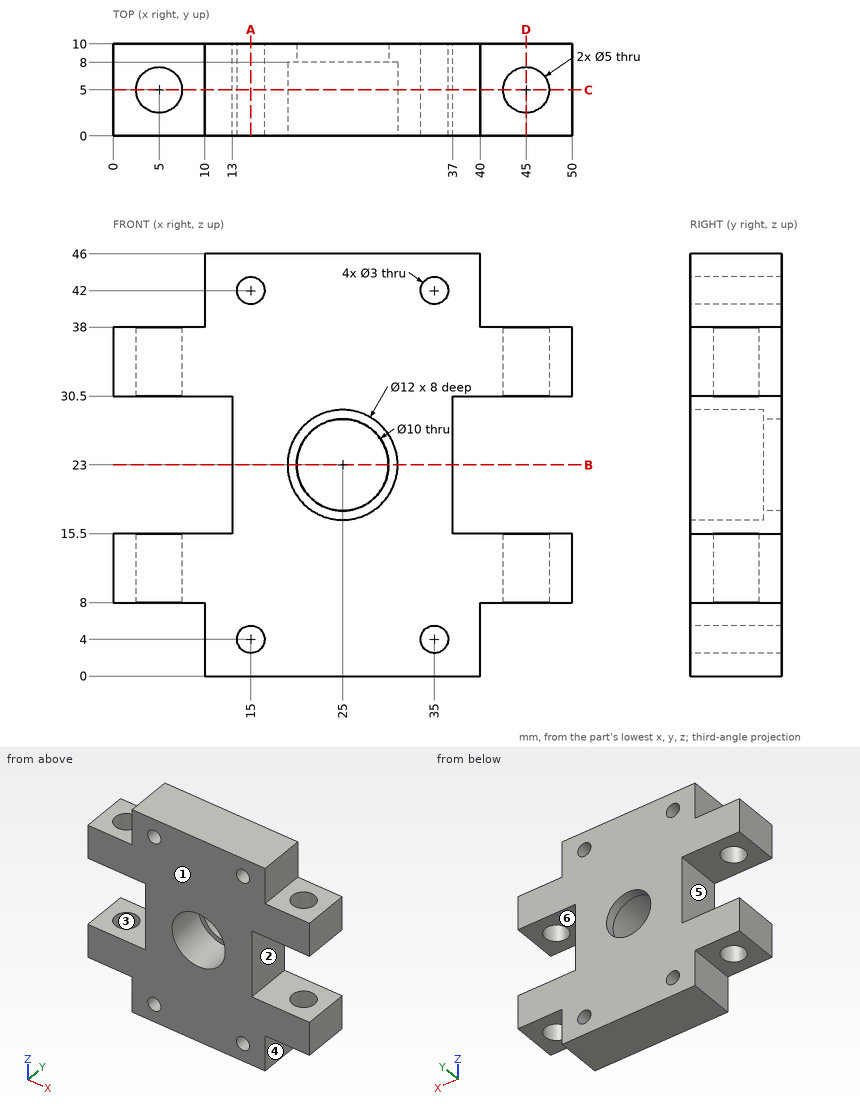
Design review of the part shown in the three views and the two pictorial views. Dimensions are in mm from the part's minimum x, y and z. A direction names the side the tool comes from. Coordinates: 2 decimals unless noted, no trailing zeros. Write each loop counter-clockwise with the first axis right and the second up, starting at its lowest first coordinate (ties: lowest second). Pieces come first, ordered by that corner, then holes.
1) To check wall thickness, follow probe 1 along X at (y, z) = (5.5, 4); probe 2 along Z at (x, y) = (16, 2.5); probe 3 along Z at (x, y) = (46, 7.5). State the ranges of each line that lie inside material, in increasing order.
2) Machinability: for the marked faces 4, 5 and 6, which of the approach directions +Z, -Z, +X, -X, +Y, -Y give a long, thin tool a straight path to every point of the face, cutting with its end or side? Answer none if there is none.
3) We need section A-A on x = 15. State the section outline as (y, z) points.
4) We need section D-D on x = 45. State the section outline as (y, z) points.
5) We need section B-B on z = 23. State the section outline as (x, y) points, then the cut area to 3 significant figures.
6) We need section C-C on y = 5. Count the separate pieces of the cut face and the enclosed holes in it, then the cut area to 3 significant figures.
7) The part is to be moulded in two halves that separate along X. For the marked faces 1, 2 and 3, say which applies: pulls with the +X half, pulls with the -X half, needs draft (parallel to the pull), parting line crosses it, or undercut.
8) Clearance check with flat-ended pins moving along their axes: pin 1 Ø4 at (x, y) = (5, 5) entering from +Z; pin 2 Ø4 at (y, z) = (3.5, 40.5) entering from -X; pin 3 Ø4 at (y, z) = (5, 2.5) entering from +X; pin 4 Ø5 at (y, z) = (7, 26) entering from -X. State where each tip first meets the part, or that it passes through.
Answer list:
1. probe 1: x = 10 to 13.5, 16.5 to 33.5, 36.5 to 40
1. probe 2: z = 0 to 2.88, 5.12 to 40.88, 43.12 to 46
1. probe 3: z = 8 to 15.5, 30.5 to 38
2. face 4: -Z, +X, +Y, -Y
2. face 5: -X, +Y, -Y
2. face 6: +X, +Y, -Y
3. outline: (0, 0) - (10, 0) - (10, 2.5) - (0, 2.5) - close; (0, 5.5) - (10, 5.5) - (10, 40.5) - (0, 40.5) - close; (0, 43.5) - (10, 43.5) - (10, 46) - (0, 46) - close
4. outline: (0, 8) - (2.5, 8) - (2.5, 15.5) - (0, 15.5) - close; (0, 30.5) - (2.5, 30.5) - (2.5, 38) - (0, 38) - close; (7.5, 8) - (10, 8) - (10, 15.5) - (7.5, 15.5) - close; (7.5, 30.5) - (10, 30.5) - (10, 38) - (7.5, 38) - close
5. outline: (13, 0) - (19, 0) - (19, 8) - (20, 8) - (20, 10) - (13, 10) - close; (30, 8) - (31, 8) - (31, 0) - (37, 0) - (37, 10) - (30, 10) - close
5. area: 124 mm2
6. separate pieces: 5
6. enclosed holes: 5
6. area: 1,300 mm2
7. face 1: needs draft
7. face 2: pulls with the +X half
7. face 3: undercut
8. pin 1: passes through
8. pin 2: stops at x = 10
8. pin 3: stops at x = 40
8. pin 4: stops at x = 13
